```python
from build123d import *

# Parameters (mm, degrees)
EXTRUDE_1_DEPTH = 5


with BuildPart() as part:
    # Model → 凸台-拉伸1 (new body)
    with BuildSketch(Plane.XY):
        with BuildLine():
            Line((43.845523177, -177.492582663), (538.81027344, -165.856176204))
            Line((538.81027344, -165.856176204), (538.81027344, -159.776195336))
            Line((538.81027344, -159.776195336), (536.81027344, -159.776195336))
            Line((536.81027344, -159.776195336), (508.460943442, -160.297194912))
            Line((508.460943442, -160.297194912), (506.460943442, -160.297194912))
            Line((506.460943442, -160.297194912), (423.796625507, -162.048616282))
            Line((423.796625507, -162.048616282), (421.796625507, -162.048616282))
            Line((421.796625507, -162.048616282), (332.810549536, -163.795959439))
            Line((332.810549536, -163.795959439), (330.810549536, -163.795959439))
            Line((330.810549536, -163.795959439), (314.810549536, -164.194907743))
            Line((314.810549536, -164.194907743), (312.810549536, -164.194907743))
            Line((312.810549536, -164.194907743), (214.560628282, -166.204763766))
            Line((214.560628282, -166.204763766), (212.591381202, -166.204763766))
            ThreePointArc((212.591381202, -166.204763766), (212.560629898, -166.204921378), (212.529881824, -166.205394195))
            Line((212.529881824, -166.205394195), (124.560628282, -168.009124705))
            Line((124.560628282, -168.009124705), (122.560628282, -168.009124705))
            Line((122.560628282, -168.009124705), (72.913804388, -168.993411369))
            Line((72.913804388, -168.993411369), (45.043435184, -168.993411369))
            Line((45.043435184, -168.993411369), (43.780250092, -166.49051255))
            Line((43.780250092, -166.49051255), (43.775013962, -168.993411369))
            Line((43.775013962, -168.993411369), (17.81027344, -168.993411369))
            Line((17.81027344, -168.993411369), (-8.154467083, -168.993411369))
            Line((-8.154467083, -168.993411369), (-8.159703213, -166.49051255))
            Line((-8.159703213, -166.49051255), (-9.422888304, -168.993411369))
            Line((-9.422888304, -168.993411369), (-37.293257509, -168.993411369))
            Line((-37.293257509, -168.993411369), (-86.940081403, -168.009124705))
            Line((-86.940081403, -168.009124705), (-88.940081403, -168.009124705))
            Line((-88.940081403, -168.009124705), (-176.909334945, -166.205394195))
            ThreePointArc((-176.909334945, -166.205394195), (-176.940083018, -166.204921378), (-176.970834323, -166.204763766))
            Line((-176.970834323, -166.204763766), (-178.940081403, -166.204763766))
            Line((-178.940081403, -166.204763766), (-277.190002657, -164.194907743))
            Line((-277.190002657, -164.194907743), (-279.190002657, -164.194907743))
            Line((-279.190002657, -164.194907743), (-295.190002657, -163.795959439))
            Line((-295.190002657, -163.795959439), (-297.190002657, -163.795959439))
            Line((-297.190002657, -163.795959439), (-386.176078628, -162.048616282))
            Line((-386.176078628, -162.048616282), (-388.176078628, -162.048616282))
            Line((-388.176078628, -162.048616282), (-470.840396563, -160.297194912))
            Line((-470.840396563, -160.297194912), (-472.840396563, -160.297194912))
            Line((-472.840396563, -160.297194912), (-501.18972656, -159.776195336))
            Line((-501.18972656, -159.776195336), (-503.18972656, -159.776195336))
            Line((-503.18972656, -159.776195336), (-503.18972656, -165.856176204))
            Line((-503.18972656, -165.856176204), (-8.224976298, -177.492582663))
            ThreePointArc((-8.224976298, -177.492582663), (-8.189724125, -177.493204186), (-8.154467083, -177.493411369))
            Line((-8.154467083, -177.493411369), (17.81027344, -177.493411369))
            Line((17.81027344, -177.493411369), (43.775013962, -177.493411369))
            ThreePointArc((43.775013962, -177.493411369), (43.810271005, -177.493204186), (43.845523177, -177.492582663))
        make_face()
    extrude(amount=EXTRUDE_1_DEPTH)


solid = part.part
```
Could you check a few things on this model? Use its own coordinates, in mm. Give positions to 0.01 mm unless a question says otherwise; leave off trailing zeros. Loops run counter-clockwise (first coordinate to the right, second up) from the corner with the lowest first, then second, coordinate; pieces in that order, holes last. Notation, with made-up numbers: (17, -6) - (28, -6) arc R25 cw to (28, 14) - close; hole circle Ø8 at (56, 75.5). An arc over 180 degrees is marked (long way). Answer in a Markdown table with one row per item. Add a question column.
Q1. Please list where these lines run through material, in increasing order: L1, parallel to Y at x = 62.5, z = 2.1; L2, parallel to Y at x = 63.5, z = 1.7. Write a range as from..to.
Q2. If we section it at A-A (x = 1): List the corners of the cut face in (y, z) for me, plus the area to 3 significant figures.
Q3. If we section it at B-B (y = -174.75): List the corners of the cut face in (x, z) for me.
Q4. For pin 1 (1 mm diameter, centred on x = 314, z = 2.5, fed in from +Y); pin 2 (1 mm diameter, centred on x = -177.5, z = 3, fed in from +Y); pin 3 (1.6 mm diameter, centred on x = -88, z = 2, fed in from +Y), each with a flat end and sliding along its axis, tell me the tip position at first contact or that it passes through.
The answers:
| question | item | result |
|---|---|---|
| 1 | L1 | y = -177.05..-168.99 |
| 1 | L2 | y = -177.03..-168.99 |
| 2 | outline | (-177.49, 0) - (-168.99, 0) - (-168.99, 5) - (-177.49, 5) - close |
| 2 | area | 42.5 mm^2 |
| 3 | outline | (-124.88, 0) - (160.5, 0) - (160.5, 5) - (-124.88, 5) - close |
| 4 | pin 1 | stops at y = -164.19 |
| 4 | pin 2 | stops at y = -166.2 |
| 4 | pin 3 | stops at y = -168.01 |
